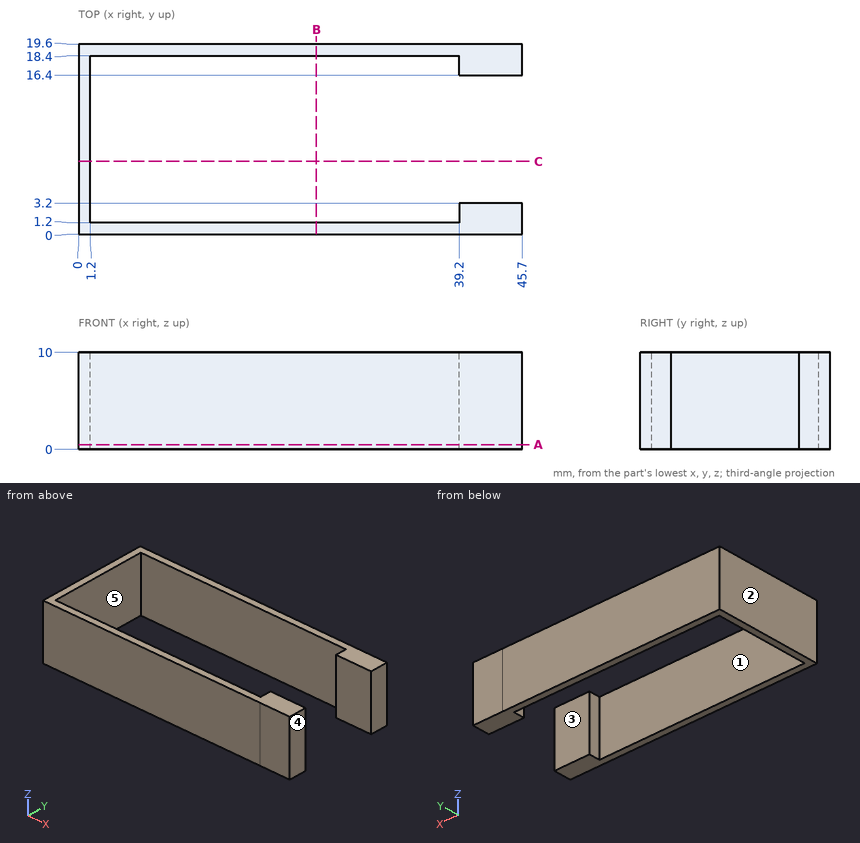
Design review of the part shown in the three views and the two pictorial views. Dimensions are in mm from the part's minimum x, y and z. A direction names the side the tool comes from. Round coordinates to 2 decimals unless told otherwise and drop trailing zeros. Loops run counter-clockwise (first coordinate to the right, second up) from the corner with the lowest first, then second, coordinate; pieces in that order, holes last. Notation, with made-up numbers: M 85,-33 L 130,-33 A14 ccw 130,-13 Z; hole C -25,28 d4. An arc over 180 degrees is marked long. Answer as a JSON object with one key per item and string values.
Item 1: Wall thickness on L1, parallel to Y at x = 11.5, z = 9.5; L2, parallel to X at y = 2.5, z = 7.25; L3, parallel to Y at x = 41, z = 7.25: over which ranges is each line inside the solid? List them lowest first. Write a range as from..to.
Answer sheet:
{"L1": "y = 0..1.2, 18.4..19.6", "L2": "x = 0..1.2, 39.2..45.7", "L3": "y = 0..3.2, 16.4..19.6"}
Item 2: We need section B-B on x = 24.5. Give the boundary of the cut face in (y, z), and give its area (3 significant figures).
Answer sheet:
{"outline": "M 0,0 L 1.2,0 L 1.2,10 L 0,10 Z; M 18.4,0 L 19.6,0 L 19.6,10 L 18.4,10 Z", "area": "24.0 mm^2"}
Item 3: We need section C-C on y = 7.5. Give the boundary of the cut face in (x, z), and give its area (3 significant figures).
Answer sheet:
{"outline": "M 0,0 L 1.2,0 L 1.2,10 L 0,10 Z", "area": "12.0 mm^2"}
Item 4: Clearance check with flat-ended pins moving along their axes: P1, Ø0.6, axis at y = 2.5, z = 6, coming from the -X side; P2, Ø5, axis at y = 7.5, z = 6, coming from the +X side; P3, Ø8, axis at x = 30, y = 13.5, coming from the +Z side. State where each tip first meets the part, or that it passes through.
Answer sheet:
{"P1": "stops at x = 0", "P2": "stops at x = 1.2", "P3": "passes through"}
Item 5: The part is to be moulded in two halves that separate along Y. For the marked faces 4 and 5, say which applies: pulls with the +Y half, pulls with the -Y half, needs draft (parallel to the pull), parting line crosses it, or undercut.
Answer sheet:
{"face 4": "needs draft", "face 5": "undercut"}
Item 6: Machinability: for the marked faces 1, 2 and 3, which of the approach directions +Z, -Z, +X, -X, +Y, -Y give a long, thin tool a straight path to every point of the face, cutting with its end or side? Answer none if there is none.
Answer sheet:
{"face 1": "+Z, -Z", "face 2": "+Z, -Z, -X, +Y, -Y", "face 3": "+Z, -Z, +X"}
Item 7: We need section A-A on z = 0.5. Give the boundary of the cut face in (x, y), and give its area (3 significant figures).
Answer sheet:
{"outline": "M 0,0 L 45.7,0 L 45.7,3.2 L 39.2,3.2 L 39.2,1.2 L 1.2,1.2 L 1.2,18.4 L 39.2,18.4 L 39.2,16.4 L 45.7,16.4 L 45.7,19.6 L 0,19.6 Z", "area": "156 mm^2"}
